Design review of the part built by this model. Coordinates are the model's own, in mm. A direction names the side the tool comes from. Coordinates: 2 decimals unless noted, no trailing zeros. Loops run counter-clockwise (first coordinate to the right, second up) from the corner with the lowest first, then second, coordinate; pieces in that order, holes last.
from build123d import *

# Parameters (mm, degrees)
SKETCH2_R           = 45.59
SKETCH2_R_2         = 44.59
BOSS_EXTRUDE3_START = 130
SKETCH4_R           = 45.59
SKETCH4_R_2         = 44.59
BOSS_EXTRUDE3_DEPTH = 130


with BuildPart() as part:
    # Sweep1: sweep along a path in Sketch1
    with BuildLine(Plane(origin=(0, 0, 0), x_dir=(1, 0, 0), z_dir=(0, 1, 0))) as sweep1_path:
        Line((0, 0), (0, 150))
        ThreePointArc((0, 150), (-20.502525317, 199.497474683), (-70, 220))
        Line((-70, 220), (-630, 220))
        ThreePointArc((-630, 220), (-679.497474683, 240.502525317), (-700, 290))
        Line((-700, 290), (-700, 470))
    # Sketch2 → Sweep1 (sweep)
    with BuildSketch(Plane.XY):
        Circle(SKETCH2_R)
        Circle(SKETCH2_R_2, mode=Mode.SUBTRACT)
    sweep(path=sweep1_path.line)

    # Sketch4 → Boss-Extrude3 (add)
    with BuildSketch(Plane(origin=(0, 0, -470), x_dir=(-1, 0, 0), z_dir=(0, 0, -1)).offset(BOSS_EXTRUDE3_START)):
        with Locations((700, 0)):
            Circle(SKETCH4_R)
        with Locations((700, 0)):
            Circle(SKETCH4_R_2, mode=Mode.SUBTRACT)
    extrude(amount=-BOSS_EXTRUDE3_DEPTH)


solid = part.part
Q1. Take a section at A-A, the plane y = 0. Write out the cut boundary in (x, z), then the cut area to 3 significant figures.
Q2. Clearance check with flat-ended pins moving along their axes: pin 1 Ø4 at (x, y) = (-542.5, 30) entering from -Z; pin 2 Ø2 at (x, y) = (-609.5, -9.5) entering from -Z; pin 3 Ø1.5 at (y, z) = (-15.5, -313.5) entering from +X. State where each tip first meets the part, or that it passes through.
Q3. Take a section at B-B, the plane x = -313. Write out the cut boundary in (y, z), then the cut area to 3 significant figures.
Q4. The part is to be moulded in two halves that separate along X. For faces 1 (the cylindrical face through (43.485, -13.694, -76.05)), 2 (the cylindrical face through (-353.92, 17.08, -261.19)), 3 (the flat face through (10, -44, 0)), say which applies: pulls with the +X half, pulls with the -X half, needs draft (parallel to the pull), parting line crosses it, or undercut.
Q5. Machinability: for faces 4 (the cylindrical face through (-9.67, 43.53, -76.05)), 5 (the flat face through (-744, -10, -600)), 6 (the cylindrical face through (-353.92, 17.461, -262.114)), which of the approach directions +Z, -Z, +X, -X, +Y, -Y give a long, thin tool a straight path to every point of the face, cutting with its end or side? Answer none if there is none.
Q6. For line 1 (X direction, y = 4, z = -513.5); line 2 (Y direction, x = 0, z = -40); line 3 (X direction, y = 0, z = -416), list the stretches that pass through material, from the lowest coordinate up.
Q7. Take a section at C-C, the plane z = -498. Write out the cut boundary in (x, y), then the cut area to 3 significant figures.
Entries:
1. outline: (-745.59, -600) - (-744.59, -600) - (-744.59, -290) arc R114.59 cw to (-630, -175.41) - (-70, -175.41) arc R25.41 ccw to (-44.59, -150) - (-44.59, 0) - (-45.59, 0) - (-45.59, -150) arc R24.41 cw to (-70, -174.41) - (-630, -174.41) arc R115.59 ccw to (-745.59, -290) - close; (-655.41, -600) - (-654.41, -600) - (-654.41, -290) arc R24.41 cw to (-630, -265.59) - (-70, -265.59) arc R115.59 ccw to (45.59, -150) - (45.59, 0) - (44.59, 0) - (44.59, -150) arc R114.59 cw to (-70, -264.59) - (-630, -264.59) arc R25.41 ccw to (-655.41, -290) - close
1. area: 2,480 mm2
2. pin 1: stops at z = -255.98
2. pin 2: stops at z = -264.79
2. pin 3: stops at x = -656.86
3. outline: circle Ø91.18 at (0, -220); hole circle Ø89.18 at (0, -220)
3. area: 283 mm2
4. face 1: parting line crosses it
4. face 2: undercut
4. face 3: needs draft
5. face 4: +Z
5. face 5: -Z, +X, -X, +Y, -Y
5. face 6: none
6. line 1: x = -745.41 to -744.41, -655.59 to -654.59
6. line 2: y = -45.59 to -44.59, 44.59 to 45.59
6. line 3: x = -745.59 to -744.59, -655.41 to -654.41
7. outline: circle Ø91.18 at (-700, 0); hole circle Ø89.18 at (-700, 0)
7. area: 283 mm2
